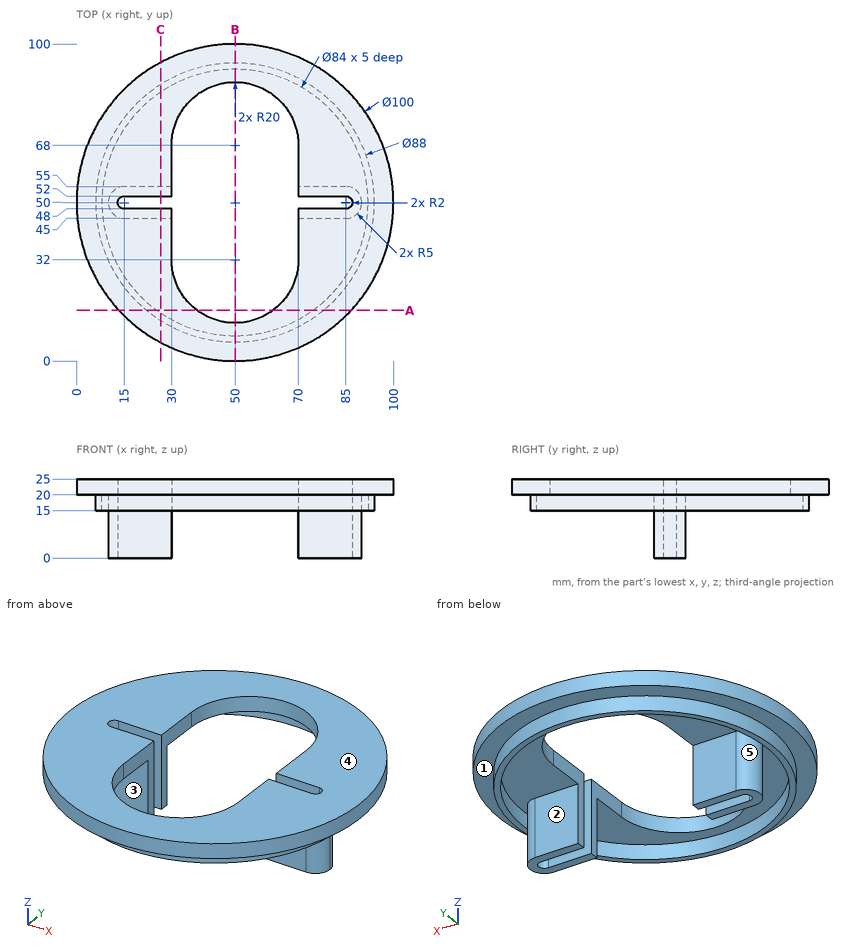
Can you work these out from the drawing? Everything is in mm from the part's minimum corner. A direction names the side the tool comes from. Give positions to 0.01 mm unless a question says otherwise; leave off trailing zeros. Write each loop counter-clockwise with the first axis right and the second up, starting at its lowest first coordinate (ties: lowest second). Pieces come first, ordered by that corner, then holes. Notation, with made-up numbers: M 30,-31.5 L 59,-31.5 A23 cw 59,-12.5 Z; hole C -10.75,59 d8. An arc over 180 degrees is marked long. Answer in a Markdown table with one row per item. Add a question column.
Item 1: Imagine slicing it at C-C, the plane x = 26.5. Write out the boundary of the cut face in (y, z), plus the area to 3 significant figures.
Item 2: Imagine slicing it at A-A, the plane y = 16. Write out the boundary of the cut face in (x, z), plus the area to 3 significant figures.
Item 3: Imagine slicing it at B-B, the plane x = 50. Write out the boundary of the cut face in (y, z), plus the area to 3 significant figures.
Item 4: We'd pull the mould along Y, two halves only. Please class the marked faces 1, 2 and 3: released by +Y, released by -Y, zero draft, split by the parting line, or undercut.
Item 5: For pin 1 Ø2 at (x, z) = (29.5, 10) entering from +Y; pin 2 Ø5 at (y, z) = (64, 11) entering from +X; pin 3 Ø1 at (y, z) = (85, 20) entering from +X; pin 4 Ø12 at (x, z) = (21, 16.5) entering from -Y, each with a flat end and sliding along its axis, tell me the tip position at first contact or that it passes through.
Item 6: Please list where these lines run through material, in increasing order: L1, parallel to Y at x = 50, z = 18.8; L2, parallel to Y at x = 11.5, z = 19.25; L3, parallel to Y at x = 24, z = 2.25.
Item 7: On a 3-axis mill with a long thin cutter (end or side, diameter ignored), from which of +Z, -Z, +X, -X, +Y, -Y can I reach the whole of each face in a straight line? I mean the marked faces 4 and 5. Say none if no direction works.
Evaluation:
| question | item | result |
|---|---|---|
| 1 | outline | M 5.87,20 L 12.8,20 L 12.8,15 L 15.19,15 L 15.19,20 L 45,20 L 45,0 L 48,0 L 48,25 L 5.87,25 Z; M 52,0 L 55,0 L 55,20 L 84.81,20 L 84.81,15 L 87.2,15 L 87.2,20 L 94.13,20 L 94.13,25 L 52,25 Z |
| 1 | area | 565 mm² |
| 2 | outline | M 13.34,20 L 22.07,20 L 22.07,15 L 25.34,15 L 25.34,20 L 38,20 L 38,25 L 13.34,25 Z; M 62,20 L 74.66,20 L 74.66,15 L 77.93,15 L 77.93,20 L 86.66,20 L 86.66,25 L 62,25 Z |
| 2 | area | 279 mm² |
| 3 | outline | M 0,20 L 6,20 L 6,15 L 8,15 L 8,20 L 12,20 L 12,25 L 0,25 Z; M 88,20 L 92,20 L 92,15 L 94,15 L 94,20 L 100,20 L 100,25 L 88,25 Z |
| 3 | area | 140 mm² |
| 4 | face 1 | zero draft |
| 4 | face 2 | undercut |
| 4 | face 3 | undercut |
| 5 | pin 1 | stops at y = 55 |
| 5 | pin 2 | passes through |
| 5 | pin 3 | stops at x = 86.19 |
| 5 | pin 4 | stops at y = 6.21 |
| 6 | L1 | y = 6 to 8, 92 to 94 |
| 6 | L2 | y = 28.7 to 33.21, 46.43 to 53.57, 66.79 to 71.3 |
| 6 | L3 | y = 45 to 48, 52 to 55 |
| 7 | face 4 | +Z, +X, -X, +Y, -Y |
| 7 | face 5 | -Z |
